Here's how the part is built. I have some questions about the finished solid (model axes, mm). Face numbers are marked on the shaded views. A direction names the side the tool comes from. Round coordinates to 2 decimals unless told otherwise and drop trailing zeros. Order: outer loops, then holes, each group sorted by start corner. A loop starts at its lowest first (then second) coordinate and runs counter-clockwise, first axis right, second up.
Autodesk Inventor part; units mm, degrees
ref_plane "YZ Plane" through (0, 0, 0) normal (1, 0, 0) x (0, 1, 0)
ref_plane "XZ Plane" through (0, 0, 0) normal (0, 1, 0) x (-1, 0, 0)
ref_plane "XY Plane" through (0, 0, 0) normal (0, 0, 1) x (1, 0, 0)
sketch "Sketch1" plane through (0, 0, 0) normal (0, 0, 1) x (1, 0, 0)
  line L0 (-19.6971, 0) -> (73.2828, 0) construction
  line L1 (0, 49.2828) -> (0, -15.6971) construction
  line L2 (-6, 40) -> (-6, -4)
  line L3 (-4, -6) -> (60, -6)
  line L4 (60, -6) -> (60, -2)
  line L5 (60, -2) -> (0, -2)
  line L6 (-2, 0) -> (-2, 40)
  line L7 (-2, 40) -> (-6, 40)
  arc A0 (-2, 0) -> (0, -2) centre (0, 0) ccw
  arc A1 (-6, -4) -> (-4, -6) centre (-4, -4) ccw
  dimension "d0" = 2
  dimension "d1" = 4
  dimension "d2" = 4
  dimension "d3" = 40
  dimension "d5" = 60
extrude "Extrusion1" add sketch "Sketch1" along normal mid plane 38
sketch "Sketch2" plane through (-2, 0, 19) normal (1, 0, 0) x (0, 0, -1)
  line L0 (0, 40) -> (38, 40) construction
  line L1 (0, 0) -> (0, 40) construction
  line L2 (38, 0) -> (0, 0) construction
  line L3 (38, 40) -> (38, 0) construction
  line L4 (0, 0) -> (0, 40) construction
  line L5 (0, 20) -> (38, 20) construction
  line L6 (19, 0) -> (19, 40) construction
  line L7 (0, 40) -> (38, 40) construction
  circle A0 centre (19, 20) radius 20 construction
  point P0 (33.1421, 5.8579)
  point P1 (33.1421, 34.1421)
  point P2 (4.8579, 5.8579)
  point P3 (4.8579, 34.1421)
  dimension "d17" = 40
  dimension "d18" = 28.2843
  dimension "d19" = 28.2843
hole "Hole1" at (-2, 5.8579, -14.1421) at (-2, 34.1421, -14.1421) at (-2, 5.8579, 14.1421) at (-2, 34.1421, 14.1421) direction (-1, 0, 0) diameter 5.5 end through all
sketch "Sketch3" plane through (-4, -6, 19) normal (0, -1, 0) x (1, 0, 0)
  line L0 (64, -38) -> (64, 0) construction
  line L1 (0, 0) -> (64, 0) construction
  line L2 (0, -38) -> (0, 0) construction
  line L3 (64, -38) -> (0, -38) construction
  line L4 (64, -19) -> (0, -19) construction
  line L5 (0, -38) -> (0, 0) construction
  line L6 (64, 0) -> (4, 0) construction
  line L7 (4, -38) -> (64, -38) construction
  line L8 (54, -11.5) -> (14, -11.5) construction
  line L9 (14, -11.5) -> (14, -26.5) construction
  line L10 (14, -26.5) -> (54, -26.5) construction
  line L11 (54, -26.5) -> (54, -11.5) construction
  line L12 (64, -38) -> (0, -38) construction
  line L13 (2, 0) -> (-2, 0) construction
  line L14 (4, -38) -> (4, 0) construction
  line L15 (34, 0) -> (34, -38) construction
  point P0 (4, -19)
  dimension "d20" = 15
  dimension "d21" = 40
hole "Hole2" at (50, -6, 7.5) at (50, -6, -7.5) at (10, -6, -7.5) at (10, -6, 7.5) direction (0, 1, 0) diameter 5.5 end through all
properties part number "L_connector_actuators_endeffector"
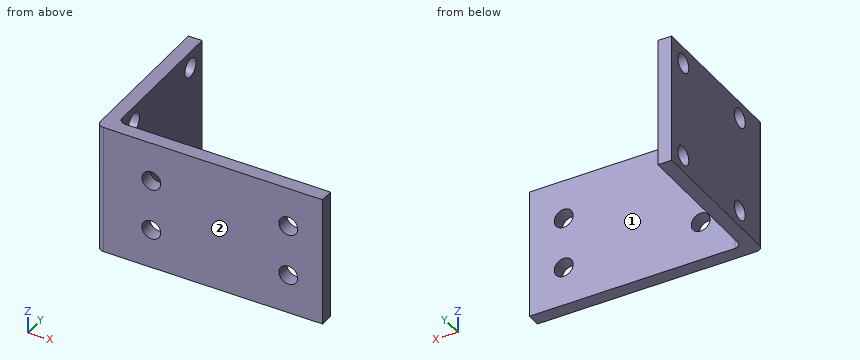
1) I'm going to push flat-ended pins straight in: pin 1 (12 mm diameter, centred on y = 26.5, z = -7.5, fed in from +X); pin 2 (4 mm diameter, centred on x = 53, z = 8.5, fed in from +Y). Where does each tip first touch, or does it pass through?
2) If we section it at A-A (z = -7.5): Write out the boundary of the cut face in (x, y).
3) If we section it at B-B (x = 50): Write out the boundary of the cut face in (y, z), plus the area to 3 significant figures.
4) I need wall thicknesses on line 1 (Z direction, x = 10, y = -4.8); line 2 (X direction, y = -4.55, z = 7.5); line 3 (X direction, y = -5.2, z = 7.5). Which ranges of each line are inside material? Lowest first, please.
5) If we section it at D-D (z = 14.5): Write out the boundary of the cut face in (x, y).
6) For the marked faces 1 and 2, which set-ups out of +Z, -Z, +X, -X, +Y, -Y let a thin tool reach every point of the face, with its end or its side?
7) If we section it at C-C (y = 33): Write out the boundary of the cut face in (x, z).
Solutions:
1. pin 1: stops at x = -2
1. pin 2: stops at y = -2
2. outline: (-6, -4) arc R2 ccw to (-4, -6) - (7.25, -6) - (7.25, -2) - (0, -2) arc R2 cw to (-2, 0) - (-2, 40) - (-6, 40) - close; (12.75, -6) - (47.25, -6) - (47.25, -2) - (12.75, -2) - close; (52.75, -6) - (60, -6) - (60, -2) - (52.75, -2) - close
3. outline: (-6, -19) - (-2, -19) - (-2, -10.25) - (-6, -10.25) - close; (-6, -4.75) - (-2, -4.75) - (-2, 4.75) - (-6, 4.75) - close; (-6, 10.25) - (-2, 10.25) - (-2, 19) - (-6, 19) - close
3. area: 108 mm2
4. line 1: z = -19 to -10.25, -4.75 to 4.75, 10.25 to 19
4. line 2: x = -5.92 to 7.25, 12.75 to 47.25, 52.75 to 60
4. line 3: x = -5.6 to 7.25, 12.75 to 47.25, 52.75 to 60
5. outline: (-6, -4) arc R2 ccw to (-4, -6) - (60, -6) - (60, -2) - (0, -2) arc R2 cw to (-2, 0) - (-2, 3.13) - (-6, 3.13) - close; (-6, 8.58) - (-2, 8.58) - (-2, 31.42) - (-6, 31.42) - close; (-6, 36.87) - (-2, 36.87) - (-2, 40) - (-6, 40) - close
6. face 1: +Z, -Z, +X, +Y
6. face 2: +Z, -Z, +X, -X, -Y
7. outline: (-6, -19) - (-2, -19) - (-2, -16.64) - (-6, -16.64) - close; (-6, -11.64) - (-2, -11.64) - (-2, 11.64) - (-6, 11.64) - close; (-6, 16.64) - (-2, 16.64) - (-2, 19) - (-6, 19) - close
